The drawing under review shows one solid part. Ordinate dimensions are in mm from its lowest x, y, z. Give positions to 0.01 mm unless a question says otherwise; leave off trailing zeros. Write each loop counter-clockwise with the first axis right and the second up, starting at its lowest first coordinate (ties: lowest second). Pieces come first, ordered by that corner, then holes. Notation, with made-up numbers: (-37.5, 89.5) -> (-0.5, 89.5) arc R22 cw to (-0.5, 115.5) -> close; hole circle Ø4 at (-2.75, -11). An arc over 180 degrees is marked (long way). Use CSV: the item, a comma, the result in double quotes.
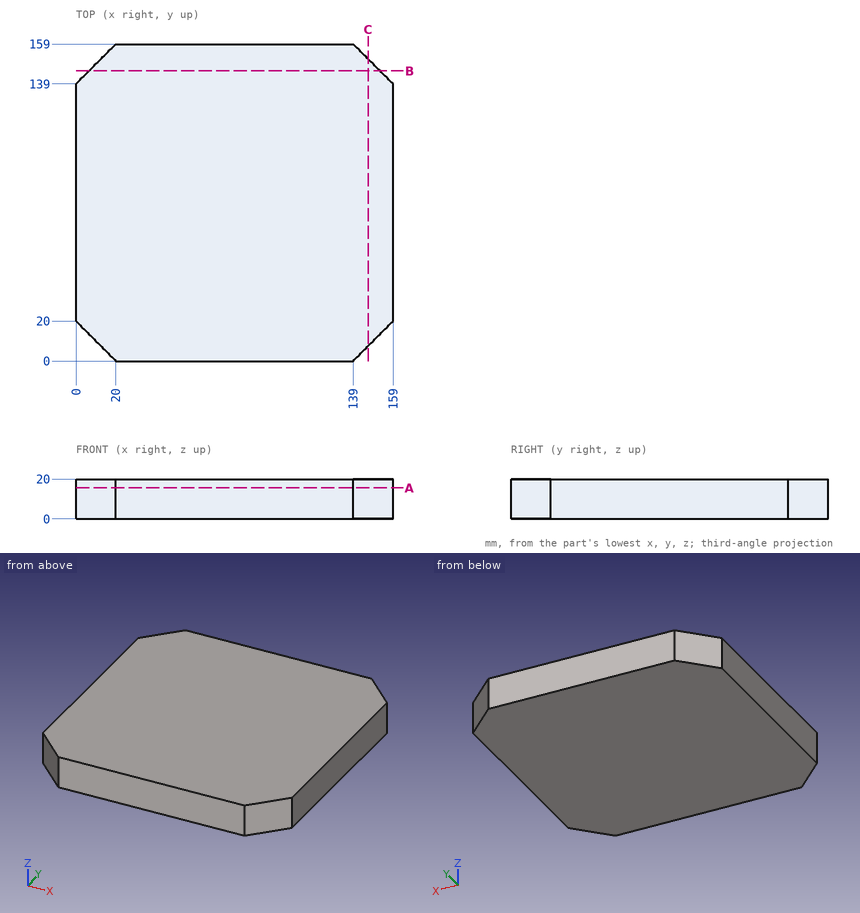
(1) For line 1 along X through (y, z) = (7, 19.25); line 2 along Y through (x, z) = (149.5, 16); line 3 along X through (y, z) = (151, 4.5), list the stretches that pass through material, from the lowest coordinate up. Write a range as [from, to].
Established:
line 1,"x = [13, 146]"
line 2,"y = [10.5, 148.5]"
line 3,"x = [12, 147]"
(2) Take a section at A-A (z = 15.5). Write out the cut boundary in (x, y), then the cut area to 3 significant figures.
Established:
outline,"(0, 20) -> (20, 0) -> (139, 0) -> (159, 20) -> (159, 139) -> (139, 159) -> (20, 159) -> (0, 139) -> close"
area,"24,500 mm2"
(3) Take a section at B-B (y = 145.5). Write out the cut boundary in (x, z), then the cut area to 3 significant figures.
Established:
outline,"(6.5, 0) -> (152.5, 0) -> (152.5, 20) -> (6.5, 20) -> close"
area,"2,920 mm2"
(4) Take a section at C-C (x = 146.5). Write out the cut boundary in (y, z).
Established:
outline,"(7.5, 0) -> (151.5, 0) -> (151.5, 20) -> (7.5, 20) -> close"
